Part model, mm, in its own coordinate system. Face numbers are marked on the shaded views. A direction names the side the tool comes from. Give positions to 0.01 mm unless a question says otherwise; leave off trailing zeros. Write each loop counter-clockwise with the first axis right and the second up, starting at its lowest first coordinate (ties: lowest second). Pieces come first, ordered by that corner, then holes. Notation, with made-up numbers: M 34.25,-38.75 L 68.25,-38.75 A12 ccw 68.25,-31.75 Z; hole C 9,-31 d9. An arc over 180 degrees is marked long. Use a Markdown table: item, result. Add a question column.
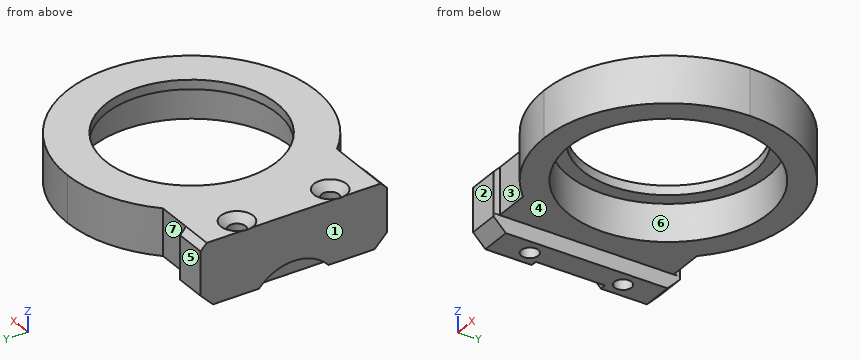
from build123d import *

# Parameters (mm, degrees)
SKETCH1_W                                       = 80
SKETCH1_H                                       = 80
BOSS_EXTRUDE1_DEPTH                             = 15
SKETCH2_R                                       = 32
CUT_EXTRUDE2_DEPTH                              = 16
SKETCH3_R                                       = 32
SKETCH3_R_2                                     = 27.5
BOSS_EXTRUDE2_DEPTH                             = 3
FILLET1_R                                       = 10
SKETCH5_W                                       = 10
SKETCH5_H                                       = 60
BOSS_EXTRUDE3_DEPTH                             = 20
SKETCH6_R                                       = 2.5
CUT_EXTRUDE3_DEPTH                              = 21
CHAMFER1_SIZE                                   = 2
CSK_FOR_M5_FLAT_HEAD_MACHINE_SCREW2_D           = 5.5
CSK_FOR_M5_FLAT_HEAD_MACHINE_SCREW2_CSINK_D     = 10.4
CSK_FOR_M5_FLAT_HEAD_MACHINE_SCREW2_CSINK_ANGLE = 90
CHAMFER2_SIZE                                   = 4
SKETCH11_R                                      = 15
CUT_EXTRUDE4_DEPTH                              = 2
CUT_EXTRUDE7_DEPTH                              = 21


with BuildPart() as part:
    # Sketch1 → Boss-Extrude1 (new body)
    with BuildSketch(Plane.XY):
        with Locations((40, 40)):
            Rectangle(SKETCH1_W, SKETCH1_H)
    extrude(amount=BOSS_EXTRUDE1_DEPTH)

    # Sketch2 → Cut-Extrude2 (cut, through all)
    with BuildSketch(Plane.XY.offset(15)):
        with Locations((40, 40)):
            Circle(SKETCH2_R)
    extrude(amount=-CUT_EXTRUDE2_DEPTH, mode=Mode.SUBTRACT)

    # Sketch3 → Boss-Extrude2 (add)
    with BuildSketch(Plane.XY.offset(15)):
        with Locations((40, 40)):
            Circle(SKETCH3_R)
        with Locations((40, 40)):
            Circle(SKETCH3_R_2, mode=Mode.SUBTRACT)
    extrude(amount=-BOSS_EXTRUDE2_DEPTH)

    # Fillet1
    fillet1_edges = [part.edges().sort_by_distance(p)[0] for p in [
        (0, 80, 7.5),
        (80, 80, 7.5),
        (80, 0, 7.5),
        (0, 0, 7.5),
    ]]
    fillet(fillet1_edges, radius=FILLET1_R)

    # Sketch5 → Boss-Extrude3 (add)
    with BuildSketch(Plane.XY.offset(15)):
        with Locations((-5, 40)):
            Rectangle(SKETCH5_W, SKETCH5_H)
    extrude(amount=-BOSS_EXTRUDE3_DEPTH)

    # Sketch6 → Cut-Extrude3 (cut, through all)
    with BuildSketch(Plane.XY.offset(15)):
        with Locations((-5, 55)):
            Circle(SKETCH6_R)
        with Locations((-5, 25)):
            Circle(SKETCH6_R)
    extrude(amount=-CUT_EXTRUDE3_DEPTH, mode=Mode.SUBTRACT)

    # Chamfer1
    chamfer1_edges = [part.edges().sort_by_distance(p)[0] for p in [
        (-5, 70, 15),
        (-5, 10, 15),
    ]]
    chamfer(chamfer1_edges, length=CHAMFER1_SIZE)

    # CSK for M5 Flat Head Machine Screw2 (through all)
    with Locations(Plane.XY.offset(15)):
        with Locations((-5, 55), (-5, 25)):
            CounterSinkHole(CSK_FOR_M5_FLAT_HEAD_MACHINE_SCREW2_D / 2, CSK_FOR_M5_FLAT_HEAD_MACHINE_SCREW2_CSINK_D / 2, counter_sink_angle=CSK_FOR_M5_FLAT_HEAD_MACHINE_SCREW2_CSINK_ANGLE)

    # Chamfer2
    chamfer2_edges = [part.edges().sort_by_distance(p)[0] for p in [
        (-5, 10, -5),
        (-5, 70, -5),
    ]]
    chamfer(chamfer2_edges, length=CHAMFER2_SIZE)

    # Sketch11 → Cut-Extrude4 (cut)
    with BuildSketch(Plane.ZY.offset(10)):
        with Locations((-15, 40)):
            Circle(SKETCH11_R)
    extrude(amount=-CUT_EXTRUDE4_DEPTH, mode=Mode.SUBTRACT)

    # Sketch12 → Cut-Extrude7 (cut, through all)
    with BuildSketch(Plane.XY.offset(15)):
        with BuildLine():
            Line((11.434286286, 12), (0.202041029, 12))
            ThreePointArc((0.202041029, 12), (0.05063847, 11.00508962), (0, 10))
            ThreePointArc((0, 10), (2.928932188, 2.928932188), (10, 0))
            Line((10, 0), (40, 0))
            ThreePointArc((40, 0), (24.508066615, 3.121822171), (11.434286286, 12))
        make_face()
        with BuildLine():
            ThreePointArc((80, 40), (68.284271247, 11.715728753), (40, 0))
            Line((40, 0), (70, 0))
            ThreePointArc((70, 0), (77.071067812, 2.928932188), (80, 10))
            Line((80, 10), (80, 40))
        make_face()
        with BuildLine():
            ThreePointArc((40.000000226, 80), (68.284271327, 68.284271168), (80, 40))
            Line((80, 40), (80, 70))
            ThreePointArc((80, 70), (77.071067812, 77.071067812), (70, 80))
            Line((70, 80), (40.000000226, 80))
        make_face()
        with BuildLine():
            ThreePointArc((11.434286286, 68), (24.508066719, 76.878177873), (40.000000226, 80))
            Line((40.000000226, 80), (10, 80))
            ThreePointArc((10, 80), (2.928932174, 77.071067798), (0, 69.99999996))
            ThreePointArc((0, 69.99999996), (0.050638472, 68.99491036), (0.202041029, 68))
            Line((0.202041029, 68), (11.434286286, 68))
        make_face()
    extrude(amount=-CUT_EXTRUDE7_DEPTH, mode=Mode.SUBTRACT)


solid = part.part
1. Cut at D-D (y = 36). Write the cut outline in (x, z), then the cut area to 3 significant figures.
2. Cut at B-B (x = 45.5). Write the cut outline in (y, z), then the cut area to 3 significant figures.
3. Flat gauge pins, fed straight in: pin 1 (1.5 mm diameter, centred on x = 62.5, z = 7, fed in from +Y); pin 2 (3 mm diameter, centred on x = -5, z = 4.5, fed in from +Y); pin 3 (3 mm diameter, centred on y = 13, z = 8.5, fed in from +X). Where does each tip first touch, or does it go through?
4. Cut at A-A (z = 1.5). Write the cut outline in (x, y).
5. Tool access for the marked faces 4, 5, 6 and 7: list every direction of +Z, -Z, +X, -X, +Y, -Y with a clear straight run to the whole face (end or side of a thin tool).
6. Mould opens along X. For the marked faces 1, 2 and 3 say: released by +X, released by -X, zero draft, split by the parting line, or undercut.
7. Cut at C-C (y = 55). Write the cut outline in (x, z), then the cut area to 3 significant figures.
8. Drill centre lines: probe 1 along Y at (x, z) = (-5, 8.25); probe 2 along X at (y, z) = (53, 7); probe 3 along Y at (x, z) = (6.5, 10). Where is each one in solid material? Low to high. Write a range as [from, to].
A:
| question | item | result |
|---|---|---|
| 1 | outline | M -10,-0.54 L -8,-0.54 L -8,-5 L 0,-5 L 0,0 L 8.25,0 L 8.25,12 L 12.79,12 L 12.79,15 L -10,15 Z; M 67.21,12 L 71.75,12 L 71.75,0 L 79.8,0 L 79.8,15 L 67.21,15 Z |
| 1 | area | 463 mm² |
| 2 | outline | M 0.38,0 L 8.48,0 L 8.48,12 L 13.06,12 L 13.06,15 L 0.38,15 Z; M 66.94,12 L 71.52,12 L 71.52,0 L 79.62,0 L 79.62,15 L 66.94,15 Z |
| 2 | area | 270 mm² |
| 3 | pin 1 | stops at y = 73.57 |
| 3 | pin 2 | stops at y = 70 |
| 3 | pin 3 | stops at x = 70.82 |
| 4 | outline | M -10,10 L 0,10 A10 cw 0.2,12 L 11.43,12 A40 ccw long 11.43,68 L 0.2,68 A10 cw 0,70 L -10,70 Z; hole C -5,25 d5.5; hole C -5,55 d5.5; hole C 40,40 d64 |
| 5 | face 4 | -Z, +X, +Y, -Y |
| 5 | face 5 | +Z, -Z, -X, +Y |
| 5 | face 6 | -Z |
| 5 | face 7 | +Z, -Z, +Y |
| 6 | face 1 | released by -X |
| 6 | face 2 | zero draft |
| 6 | face 3 | undercut |
| 7 | outline | M -10,-5 L -7.75,-5 L -7.75,12.55 L -10,14.8 Z; M -2.25,-5 L 0,-5 L 0,0 L 11.73,0 L 11.73,12 L 16.95,12 L 16.95,15 L 0.2,15 L -2.25,12.55 Z; M 63.05,12 L 68.27,12 L 68.27,0 L 77.08,0 L 77.08,15 L 63.05,15 Z |
| 7 | area | 424 mm² |
| 8 | probe 1 | y = [10, 22.25], [27.75, 52.25], [57.75, 70] |
| 8 | probe 2 | x = [-10, -6.89], [-3.11, 10.76], [69.24, 77.83] |
| 8 | probe 3 | y = [12, 68] |
